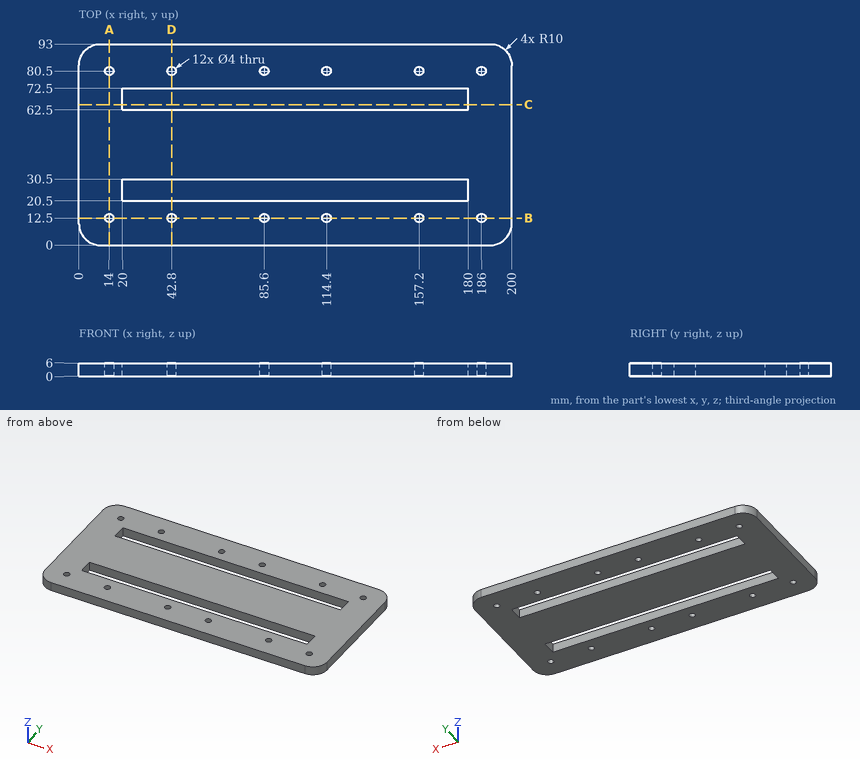
Verification items for this drawing (mm, ordinates from the low corner). Coordinates: 2 decimals unless noted, no trailing zeros. Order: outer loops, then holes, each group sorted by start corner. A loop starts at its lowest first (then second) coordinate and runs counter-clockwise, first axis right, second up. Notation, with made-up numbers: M -7.5,61 L 30.5,61 A21 cw 30.5,100 Z; hole C 7,35.5 d4. An arc over 180 degrees is marked long. Use CSV: the item, a comma, the result in double quotes.
Item 1: Cross-section at C-C on y = 65. Record the cut outline in (x, z), then the cut area to 3 significant figures.
Returned:
outline,"M 0,0 L 20,0 L 20,6 L 0,6 Z; M 180,0 L 200,0 L 200,6 L 180,6 Z"
area,"240 mm2"
Item 2: Thickness scan on line 1 along Y through (x, z) = (102, 4.2); line 2 along Y through (x, z) = (186, 1.8); line 3 along Y through (x, z) = (85.6, 4.45). Record the ranges inside material, lowest first.
Returned:
line 1,"y = 0 to 20.5, 30.5 to 62.5, 72.5 to 93"
line 2,"y = 0 to 10.5, 14.5 to 78.5, 82.5 to 93"
line 3,"y = 0 to 10.5, 14.5 to 20.5, 30.5 to 62.5, 72.5 to 78.5, 82.5 to 93"
Item 3: Gauge pin test, flat ends, axial feed: pin 1 Ø4.5 at (x, y) = (157.2, 12.5) entering from +Z; pin 2 Ø3.5 at (x, y) = (14, 12.5) entering from +Z. Record the tip position at first contact, or that the pin passes through.
Returned:
pin 1,"stops at z = 6"
pin 2,"passes through"
Item 4: Cross-section at D-D on x = 42.8. Record the cut outline in (y, z), then the cut area to 3 significant figures.
Returned:
outline,"M 0,0 L 10.5,0 L 10.5,6 L 0,6 Z; M 14.5,0 L 20.5,0 L 20.5,6 L 14.5,6 Z; M 30.5,0 L 62.5,0 L 62.5,6 L 30.5,6 Z; M 72.5,0 L 78.5,0 L 78.5,6 L 72.5,6 Z; M 82.5,0 L 93,0 L 93,6 L 82.5,6 Z"
area,"390 mm2"
Item 5: Cross-section at B-B on y = 12.5. Record the cut outline in (x, z), then the cut area to 3 significant figures.
Returned:
outline,"M 0,0 L 12,0 L 12,6 L 0,6 Z; M 16,0 L 40.8,0 L 40.8,6 L 16,6 Z; M 44.8,0 L 83.6,0 L 83.6,6 L 44.8,6 Z; M 87.6,0 L 112.4,0 L 112.4,6 L 87.6,6 Z; M 116.4,0 L 155.2,0 L 155.2,6 L 116.4,6 Z; M 159.2,0 L 184,0 L 184,6 L 159.2,6 Z; M 188,0 L 200,0 L 200,6 L 188,6 Z"
area,"1,060 mm2"
Item 6: Cross-section at A-A on x = 14. Record the cut outline in (y, z).
Returned:
outline,"M 0,0 L 10.5,0 L 10.5,6 L 0,6 Z; M 14.5,0 L 78.5,0 L 78.5,6 L 14.5,6 Z; M 82.5,0 L 93,0 L 93,6 L 82.5,6 Z"
